Source: CAD feature listing. Evaluate the final solid. Frame: model axes, mm. Give positions to 0.01 mm unless a question says otherwise; leave off trailing zeros. Write each loop counter-clockwise with the first axis right and the second up, starting at its lowest first coordinate (ties: lowest second). Pieces come first, ordered by that corner, then holes.
```python
from build123d import *

# Parameters (mm, degrees)
F0_W          = 177.8
F0_H          = 47.6504
F1_DEPTH      = 69.85
F1_DEPTH_BACK = 6.35
F2_R          = 4.7752
F2_R_2        = 1.9812
F3_DEPTH      = 47.6514
F5_DEPTH      = 16.0528
F7_DEPTH      = 31.7246


with BuildPart() as f1:
    # F0 (on Top) → F1 (new body, two sides)
    with BuildSketch(Plane.XY) as f1_sk:
        with Locations((84.1375, 23.8252)):
            Rectangle(F0_W, F0_H)
    extrude(amount=-F1_DEPTH)
    extrude(f1_sk.sketch, amount=F1_DEPTH_BACK)

    # F2 (on Front) → F3 (cut, through all)
    with BuildSketch(Plane.XZ):
        with Locations((141.5288, -11.7856)):
            Circle(F2_R)
        with Locations((112.9538, -17.5006)):
            Circle(F2_R_2)
        with Locations((91.5416, -9.525)):
            Circle(F2_R_2)
    extrude(amount=-F3_DEPTH, mode=Mode.SUBTRACT)

    # F4 (on face) → F5 (cut)
    with BuildSketch(Plane.XY.offset(6.35)):
        with BuildLine():
            Line((131.3942, 32.60725), (87.6935, 32.60725))
            ThreePointArc((87.6935, 32.60725), (84.3259039546, 31.2123460454), (82.931, 27.84475))
            Line((82.931, 27.84475), (82.931, 19.71675))
            ThreePointArc((82.931, 19.71675), (84.3259039546, 16.3491539546), (87.6935, 14.95425))
            Line((87.6935, 14.95425), (131.3942, 14.95425))
            ThreePointArc((131.3942, 14.95425), (133.7975722402, 15.6051556468), (135.5439918032, 17.37995))
            Line((135.5439918032, 17.37995), (152.4, 17.37995))
            ThreePointArc((152.4, 17.37995), (155.7675960454, 18.7748539546), (157.1625, 22.14245))
            Line((157.1625, 22.14245), (157.1625, 25.41905))
            ThreePointArc((157.1625, 25.41905), (155.7675960454, 28.7866460454), (152.4, 30.18155))
            Line((152.4, 30.18155), (135.5439918032, 30.18155))
            ThreePointArc((135.5439918032, 30.18155), (133.7975722402, 31.9563443532), (131.3942, 32.60725))
        make_face()
    extrude(amount=-F5_DEPTH, mode=Mode.SUBTRACT)

    # F6 (on face) → F7 (cut)
    with BuildSketch(Plane.XY.offset(6.35)):
        with BuildLine():
            Line((143.1901861236, 28.50515), (136.1167005926, 28.50515))
            ThreePointArc((136.1167005926, 28.50515), (134.5364877315, 31.467947555), (131.3942, 32.6517))
            Line((131.3942, 32.6517), (87.6935, 32.6517))
            ThreePointArc((87.6935, 32.6517), (84.3259039546, 31.2567960454), (82.931, 27.8892))
            Line((82.931, 27.8892), (82.931, 19.7612))
            ThreePointArc((82.931, 19.7612), (84.3259039546, 16.3936039546), (87.6935, 14.9987))
            Line((87.6935, 14.9987), (131.3942, 14.9987))
            ThreePointArc((131.3942, 14.9987), (133.77545, 15.6367540145), (135.5186459855, 17.37995))
            Line((135.5186459855, 17.37995), (143.1937903656, 17.37995))
            ThreePointArc((143.1937903656, 17.37995), (146.5651768038, 18.7786486185), (147.9562782851, 22.1531768833))
            Line((147.9562782851, 22.1531768833), (147.9526740432, 23.7533768833))
            ThreePointArc((147.9526740432, 23.7533768833), (146.5539875051, 27.1140364382), (143.1901861236, 28.50515))
        make_face()
    extrude(amount=-F7_DEPTH, mode=Mode.SUBTRACT)


solid = f1.part
```
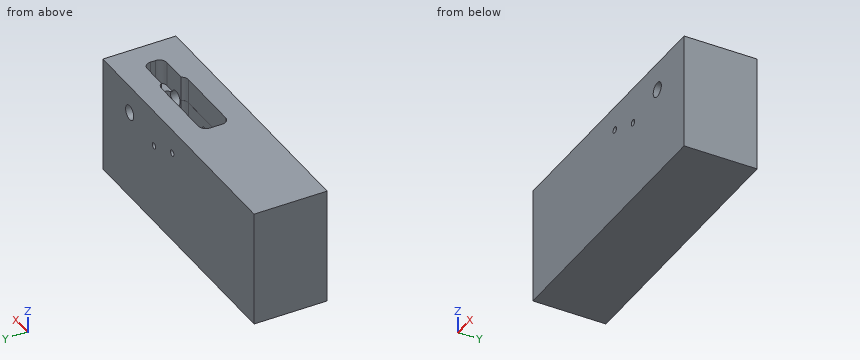
1. Pin query (flat end, axial travel): P1, Ø5.5, axis at x = 107, y = 21, coming from the +Z side. Return the tip coordinate at first contact, or that it passes through.
2. Line query: probe 1 along X at (y, z) = (23.5, -9.5); probe 2 along Y at (x, z) = (129, -16); probe 3 along Z at (x, y) = (96, 26.5). Output: solid intervals per line, ascending.
3. Section query A-A (x = 96). Return loops of the section in (y, z), plus the area to 3 significant figures.
The answers:
1. P1: stops at z = -25.37
2. probe 1: x = -4.76 to 82.93, 157.16 to 173.04
2. probe 2: y = 0 to 15, 32.65 to 47.65
2. probe 3: z = -69.85 to -25.37
3. outline: (0, -69.85) - (47.65, -69.85) - (47.65, 6.35) - (32.65, 6.35) - (32.65, -25.37) - (15, -25.37) - (15, -9.7) - (14.95, -9.7) - (14.95, 6.35) - (0, 6.35) - close
3. area: 3,070 mm2
